Source: CAD feature listing. Evaluate the final solid. Frame: model axes, mm. A direction names the side the tool comes from. Give positions to 0.01 mm unless a question says otherwise; leave off trailing zeros. Order: outer loops, then holes, each group sorted by start corner. A loop starts at its lowest first (then second) coordinate and runs counter-clockwise, first axis right, second up. Notation, with made-up numbers: (36.5, 45.25) -> (78.5, 45.25) arc R37 ccw to (78.5, 82.25) -> close; hole circle Ø10 at (20.25, 53). An arc over 180 degrees is marked (long way). Use one line per item in the form item = value. Start each with the question number.
from build123d import *

# Parameters (mm, degrees)
BOSS_EXTRU_1_DEPTH      = 3.175
SKETCH1_R               = 4.7625
CUT_EXTRUDE1_DEPTH      = 6.35
ENL_V_MAT_EXTRU_1_DEPTH = 6.35
ESQUISSE3_W             = 5.715
ESQUISSE3_H             = 45
ENL_V_MAT_EXTRU_2_DEPTH = 6.35
ENL_V_MAT_EXTRU_3_REACH = 308.007
ESQUISSE5_R             = 1.83
ENL_V_MAT_EXTRU_4_REACH = 308.007
SKETCH3_W               = 25
SKETCH3_H               = 6.35
BOSS_EXTRUDE2_DEPTH     = 6.35


with BuildPart() as part:
    # Esquisse1 → Boss.-Extru.1 (new, symmetric)
    with BuildSketch(Plane.XY):
        Polygon((-20, 300), (20, 300), (20, 80), (26.35, 80), (60, 0), (-60, 0), (-26.35, 80), (-20, 80), align=None)
    extrude(amount=BOSS_EXTRU_1_DEPTH, both=True)

    # Sketch1 → Cut-Extrude1 (cut)
    with BuildSketch(Plane.XY.offset(3.175)):
        with Locations((0, 275)):
            Circle(SKETCH1_R)
        with Locations((0, 225)):
            Circle(SKETCH1_R)
    extrude(amount=-CUT_EXTRUDE1_DEPTH, mode=Mode.SUBTRACT)

    # Esquisse2 → Enlèv. mat.-Extru.1 (cut)
    with BuildSketch(Plane.XY.offset(3.175)):
        with BuildLine():
            Line((-12.5, 0), (12.5, 0))
            add(Edge.make_bspline(
                [(12.5, 0), (12.5, 10), (0, 10), (-12.5, 10), (-12.5, 0)],
                knots=[0, 0, 0, 1.570796327, 1.570796327, 3.141592654, 3.141592654, 3.141592654], degree=2, weights=[1, 0.707106781, 1, 0.707106781, 1]))
        make_face()
    extrude(amount=-ENL_V_MAT_EXTRU_1_DEPTH, mode=Mode.SUBTRACT)

    # Esquisse3 → Enlèv. mat.-Extru.2 (cut)
    with BuildSketch(Plane.XY.offset(3.175)):
        with Locations((0.3175, 22.5)):
            Rectangle(ESQUISSE3_W, ESQUISSE3_H)
    extrude(amount=-ENL_V_MAT_EXTRU_2_DEPTH, mode=Mode.SUBTRACT)

    # Esquisse5 → Enlèv. mat.-Extru.3 (cut, up to next)
    with BuildSketch(Plane(origin=(0, 0, -3.175), x_dir=(-1, 0, 0), z_dir=(0, 0, -1)), mode=Mode.PRIVATE) as enl_v_mat_extru_3_sk1:
        with Locations((-8.5, 46)):
            Circle(ESQUISSE5_R)
    enl_v_mat_extru_3_tool1 = extrude(enl_v_mat_extru_3_sk1.sketch, amount=-ENL_V_MAT_EXTRU_3_REACH, mode=Mode.PRIVATE) & part.part
    # Esquisse5 → Enlèv. mat.-Extru.3 (cut, up to next)
    with BuildSketch(Plane(origin=(0, 0, -3.175), x_dir=(-1, 0, 0), z_dir=(0, 0, -1)), mode=Mode.PRIVATE) as enl_v_mat_extru_3_sk2:
        with Locations((8.5, 46)):
            Circle(ESQUISSE5_R)
    enl_v_mat_extru_3_tool2 = extrude(enl_v_mat_extru_3_sk2.sketch, amount=-ENL_V_MAT_EXTRU_3_REACH, mode=Mode.PRIVATE) & part.part
    # Esquisse5 → Enlèv. mat.-Extru.3 (cut, up to next)
    with BuildSketch(Plane(origin=(0, 0, -3.175), x_dir=(-1, 0, 0), z_dir=(0, 0, -1)), mode=Mode.PRIVATE) as enl_v_mat_extru_3_sk3:
        with Locations((8.5, 14)):
            Circle(ESQUISSE5_R)
    enl_v_mat_extru_3_tool3 = extrude(enl_v_mat_extru_3_sk3.sketch, amount=-ENL_V_MAT_EXTRU_3_REACH, mode=Mode.PRIVATE) & part.part
    # Esquisse5 → Enlèv. mat.-Extru.3 (cut, up to next)
    with BuildSketch(Plane(origin=(0, 0, -3.175), x_dir=(-1, 0, 0), z_dir=(0, 0, -1)), mode=Mode.PRIVATE) as enl_v_mat_extru_3_sk4:
        with Locations((-8.5, 14)):
            Circle(ESQUISSE5_R)
    enl_v_mat_extru_3_tool4 = extrude(enl_v_mat_extru_3_sk4.sketch, amount=-ENL_V_MAT_EXTRU_3_REACH, mode=Mode.PRIVATE) & part.part
    add(enl_v_mat_extru_3_tool1.solids().sort_by_distance((8.5, 46, -3.175))[0], mode=Mode.SUBTRACT)
    add(enl_v_mat_extru_3_tool2.solids().sort_by_distance((-8.5, 46, -3.175))[0], mode=Mode.SUBTRACT)
    add(enl_v_mat_extru_3_tool3.solids().sort_by_distance((-8.5, 14, -3.175))[0], mode=Mode.SUBTRACT)
    add(enl_v_mat_extru_3_tool4.solids().sort_by_distance((8.5, 14, -3.175))[0], mode=Mode.SUBTRACT)

    # Esquisse6 → Enlèv. mat.-Extru.4 (cut, up to next)
    with BuildSketch(Plane.XY.offset(3.175), mode=Mode.PRIVATE) as enl_v_mat_extru_4_sk1:
        with BuildLine():
            Line((-11.835, 185), (-11.835, 85))
            ThreePointArc((-11.835, 85), (-10, 83.165), (-8.165, 85))
            Line((-8.165, 85), (-8.165, 185))
            ThreePointArc((-8.165, 185), (-10, 186.835), (-11.835, 185))
        make_face()
    enl_v_mat_extru_4_tool1 = extrude(enl_v_mat_extru_4_sk1.sketch, amount=-ENL_V_MAT_EXTRU_4_REACH, mode=Mode.PRIVATE) & part.part
    # Esquisse6 → Enlèv. mat.-Extru.4 (cut, up to next)
    with BuildSketch(Plane.XY.offset(3.175), mode=Mode.PRIVATE) as enl_v_mat_extru_4_sk2:
        with BuildLine():
            Line((11.835, 185), (11.835, 85))
            ThreePointArc((11.835, 85), (10, 83.165), (8.165, 85))
            Line((8.165, 85), (8.165, 185))
            ThreePointArc((8.165, 185), (10, 186.835), (11.835, 185))
        make_face()
    enl_v_mat_extru_4_tool2 = extrude(enl_v_mat_extru_4_sk2.sketch, amount=-ENL_V_MAT_EXTRU_4_REACH, mode=Mode.PRIVATE) & part.part
    add(enl_v_mat_extru_4_tool1.solids().sort_by_distance((-10, 135, 3.175))[0], mode=Mode.SUBTRACT)
    add(enl_v_mat_extru_4_tool2.solids().sort_by_distance((10, 135, 3.175))[0], mode=Mode.SUBTRACT)

    # Sketch3 → Boss-Extrude2 (add)
    with BuildSketch(Plane(origin=(0, 0, 0), x_dir=(-1, 0, 0), z_dir=(0, -1, 0))):
        with Locations((-36.25, 0)):
            Rectangle(SKETCH3_W, SKETCH3_H)
        with Locations((36.25, 0)):
            Rectangle(SKETCH3_W, SKETCH3_H)
    extrude(amount=BOSS_EXTRUDE2_DEPTH)


solid = part.part
1) Cut plane B-B, the plane y = 88. Return the cut outline in (x, z) (3 decimals), plus the area to 3 significant figures.
2) Draft query along X for faces 6 (the face through (-48.75, -3, 0)), 7 (the face through (11.835, 136, 0)), 8 (the face through (-18, 0, 0)), 9 (the face through (1, 115, -3.175)). Return one class per face: +X half, -X half, draft (parallel to the pull), parting line (faces both ways), or undercut.
3) Material intervals for probe 1 along Y at (x, z) = (0, 1); probe 2 along X at (y, z) = (156, -1.5) (3 decimals); probe 3 along Y at (x, z) = (-8.5, 0.5), sorted ascending.
4) Pin query (flat end, axial travel): pin 1 (2 mm diameter, centred on x = 1.5, z = 1, fed in from -Y); pin 2 (10 mm diameter, centred on x = -22, y = 154, fed in from -Z) (3 decimals); pin 3 (1.9 mm diameter, centred on x = 16.5, z = -1, fed in from -Y); pin 4 (1.9 mm diameter, centred on y = -4, z = 1.5, fed in from -X). Return the tip coordinate at first contact, or that it passes through.
5) Cut plane D-D, the plane x = 52.5. Return the cut outline in (y, z) (3 decimals).
6) Cut plane C-C, the plane z = 1.25. Count the separate pieces of the cut face and the enclosed holes in it, plus the area to 3 significant figures.
7) Reachability of faces 1 (the face through (-23, 80, 0)), 2 (the face through (-11.835, 136, 0)), 3 (the face through (3.175, 27, 0)), 4 (the face through (1, 115, 3.175)), 5 (the face through (54, 0, 0)) from +Z, -Z, +X, -X, +Y, -Y: full face, straight path, thin tool, end or side. Return the list, or none.
8) Cut plane A-A, the plane y = 225. Return the cut outline in (x, z) (1 decimal), plus the area to 3 significant figures.
Output values:
q1.outline = (-20, -3.175) -> (-11.835, -3.175) -> (-11.835, 3.175) -> (-20, 3.175) -> close; (-8.165, -3.175) -> (8.165, -3.175) -> (8.165, 3.175) -> (-8.165, 3.175) -> close; (11.835, -3.175) -> (20, -3.175) -> (20, 3.175) -> (11.835, 3.175) -> close
q1.area = 207 mm^2
q2.face_6 = -X half
q2.face_7 = undercut
q2.face_8 = undercut
q2.face_9 = draft
q3.probe_1 = 45 to 220.24, 229.76 to 270.24, 279.76 to 300
q3.probe_2 = -20 to -11.835, -8.165 to 8.165, 11.835 to 20
q3.probe_3 = 7.33 to 12.17, 15.83 to 44.17, 47.83 to 83.94, 186.06 to 300
q4.pin_1 = 45
q4.pin_2 = -3.175
q4.pin_3 = 0
q4.pin_4 = -48.75
q5.outline = (0, -3.175) -> (17.831, -3.175) -> (17.831, 3.175) -> (0, 3.175) -> close
q6.separate_pieces = 1
q6.enclosed_holes = 8
q6.area = 14,700 mm^2
q7.face_1 = +Z, -Z, -X, +Y
q7.face_2 = +Z, -Z
q7.face_3 = +Z, -Z, -Y
q7.face_4 = +Z, +X, -X, +Y, -Y
q7.face_5 = +Z, -Z, +X, -Y
q8.outline = (-20, -3.2) -> (-4.8, -3.2) -> (-4.8, 3.2) -> (-20, 3.2) -> close; (4.8, -3.2) -> (20, -3.2) -> (20, 3.2) -> (4.8, 3.2) -> close
q8.area = 194 mm^2
